```python
from build123d import *

# Parameters (mm, degrees)
SKETCH1_R              = 15
BODY_DEPTH             = 5
SKETCH2_R              = 15
SKETCH2_R_2            = 10
SLEW_BEARING_LIP_DEPTH = 2.5
SKETCH3_R              = 2.5
CUT_EXTRUDE2_DEPTH     = 22.794494718
BOSS_EXTRUDE1_DEPTH    = 20
SKETCH5_R              = 1
CUT_EXTRUDE3_DEPTH     = 30.154759474


with BuildPart() as part:
    # Sketch1 → body (new body)
    with BuildSketch(Plane.XY):
        Circle(SKETCH1_R)
    extrude(amount=BODY_DEPTH)

    # Sketch2 → slew bearing lip (cut)
    with BuildSketch(Plane(origin=(0, 0, 0), x_dir=(-1, 0, 0), z_dir=(0, 0, -1))):
        Circle(SKETCH2_R)
        Circle(SKETCH2_R_2, mode=Mode.SUBTRACT)
    extrude(amount=-SLEW_BEARING_LIP_DEPTH, mode=Mode.SUBTRACT)

    # Sketch3 → Cut-Extrude2 (cut, through all)
    with BuildSketch(Plane.XY.offset(5)):
        with Locations((-5, 5)):
            Circle(SKETCH3_R)
        with Locations((5, 5)):
            Circle(SKETCH3_R)
        with Locations((5, -5)):
            Circle(SKETCH3_R)
        with Locations((-5, -5)):
            Circle(SKETCH3_R)
    extrude(amount=-CUT_EXTRUDE2_DEPTH, mode=Mode.SUBTRACT)

    # Sketch4 → Boss-Extrude1 (add)
    with BuildSketch(Plane(origin=(0, 0, 0), x_dir=(-1, 0, 0), z_dir=(0, 0, -1))):
        with BuildLine():
            Line((0.90103413, 0.1), (1.496662955, 0.1))
            ThreePointArc((1.496662955, 0.1), (-1.5, 0), (1.496662955, -0.1))
            Line((1.496662955, -0.1), (0.90103413, -0.1))
            Line((0.90103413, -0.1), (0.90103413, 0.1))
        make_face()
    extrude(amount=-BOSS_EXTRUDE1_DEPTH)

    # Sketch5 → Cut-Extrude3 (cut, through all)
    with BuildSketch(Plane(origin=(0, 0, 0), x_dir=(-1, 0, 0), z_dir=(0, 0, -1))):
        with Locations((0, 5)):
            Circle(SKETCH5_R)
        with Locations((5, 0)):
            Circle(SKETCH5_R)
        with Locations((0, -5)):
            Circle(SKETCH5_R)
        with Locations((-5, 0)):
            Circle(SKETCH5_R)
    extrude(amount=-CUT_EXTRUDE3_DEPTH, mode=Mode.SUBTRACT)


solid = part.part
```
Check sheet for the modelled part. Datum: model origin and axes. Units: mm. A direction names the side the tool comes from. Round coordinates to 2 decimals unless told otherwise and drop trailing zeros. Order: outer loops, then holes, each group sorted by start corner. A loop starts at its lowest first (then second) coordinate and runs counter-clockwise, first axis right, second up.
1) Mould release check, pull along Y, two halves, no side actions. Record for faces 1 (the cylindrical face through (1.5, 0.06, 12.4)), 2 (the flat face through (0, 0, 20)), 3 (the cylindrical face through (-2.615, -4.249, 2.535)), 4 (the cylindrical face through (0, -4, 2)): +Y half, -Y half, draft (parallel to the pull), parting line (faces both ways), or undercut.
2) Tool access check on faces 5 (the cylindrical face through (-2.615, 5.751, 2.535)), 6 (the flat face through (-10, -3, 2.5)). Record the directions out of +Z, -Z, +X, -X, +Y, -Y that give a thin tool (end or side, any length) a straight path to the whole face; none if there is none.
3) Section check D-D (y = 9.25). Record the boundary of the cut face in (x, z), and give its area (3 significant figures).
4) Section check C-C (z = 11.5). Record the boundary of the cut face in (x, y).
5) Go/stop test with flat-tipped pins: pin 1 Ø1.8 at (x, y) = (0, -5) entering from -Z; pin 2 Ø5 at (x, z) = (-2.5, 10) entering from -Y; pin 3 Ø8 at (x, y) = (-5, -5) entering from +Z; pin 4 Ø12 at (y, z) = (1.5, 17.5) entering from -X. Record where each tip stops, or that it passes through.
6) Scan lines: line 1 (Y direction, x = 0, z = 3.65); line 2 (X direction, y = -5.5, z = 4); line 3 (Z direction, x = -1.75, y = 1). Record each from-to range of solid material in increasing order.
7) Section check B-B (y = -5). Record the boundary of the cut face in (x, z), and give its area (3 significant figures).
8) Section check A-A (x = 4.5). Record the boundary of the cut face in (y, z).
Result:
1. face 1: parting line
1. face 2: draft
1. face 3: undercut
1. face 4: undercut
2. face 5: +Z, -Z
2. face 6: -Z
3. outline: (-11.81, 2.5) - (-3.8, 2.5) - (-3.8, 0) - (3.8, 0) - (3.8, 2.5) - (11.81, 2.5) - (11.81, 5) - (-11.81, 5) - close
3. area: 78.0 mm2
4. outline: (-1.5, -0.1) arc R1.5 ccw (long way) to (-1.5, 0.1) - (-0.9, 0.1) - (-0.9, -0.1) - close
5. pin 1: passes through
5. pin 2: stops at y = -1.5
5. pin 3: stops at z = 5
5. pin 4: stops at x = -1.5
6. line 1: y = -15 to -6, -4 to 4, 6 to 15
6. line 2: x = -13.96 to -7.45, -2.55 to -0.87, 0.87 to 2.55, 7.45 to 13.96
6. line 3: z = 0 to 5
7. outline: (-14.14, 2.5) - (-8.66, 2.5) - (-8.66, 0) - (-7.5, 0) - (-7.5, 5) - (-14.14, 5) - close; (-2.5, 0) - (-1, 0) - (-1, 5) - (-2.5, 5) - close; (1, 0) - (2.5, 0) - (2.5, 5) - (1, 5) - close; (7.5, 0) - (8.66, 0) - (8.66, 2.5) - (14.14, 2.5) - (14.14, 5) - (7.5, 5) - close
7. area: 54.0 mm2
8. outline: (-14.31, 2.5) - (-8.93, 2.5) - (-8.93, 0) - (-7.45, 0) - (-7.45, 5) - (-14.31, 5) - close; (-2.55, 0) - (-0.87, 0) - (-0.87, 5) - (-2.55, 5) - close; (0.87, 0) - (2.55, 0) - (2.55, 5) - (0.87, 5) - close; (7.45, 0) - (8.93, 0) - (8.93, 2.5) - (14.31, 2.5) - (14.31, 5) - (7.45, 5) - close
